The drawing under review shows one solid part. Ordinate dimensions are in mm from its lowest x, y, z. Coordinates: 2 decimals unless noted, no trailing zeros. Loops run counter-clockwise (first coordinate to the right, second up) from the corner with the lowest first, then second, coordinate; pieces in that order, holes last. Notation, with made-up numbers: M -35,-25 L -24,-25 A23 ccw -24,-4 Z; hole C 3,40.25 d5. An arc over 180 degrees is marked long. Put each result on its own line as item: value.
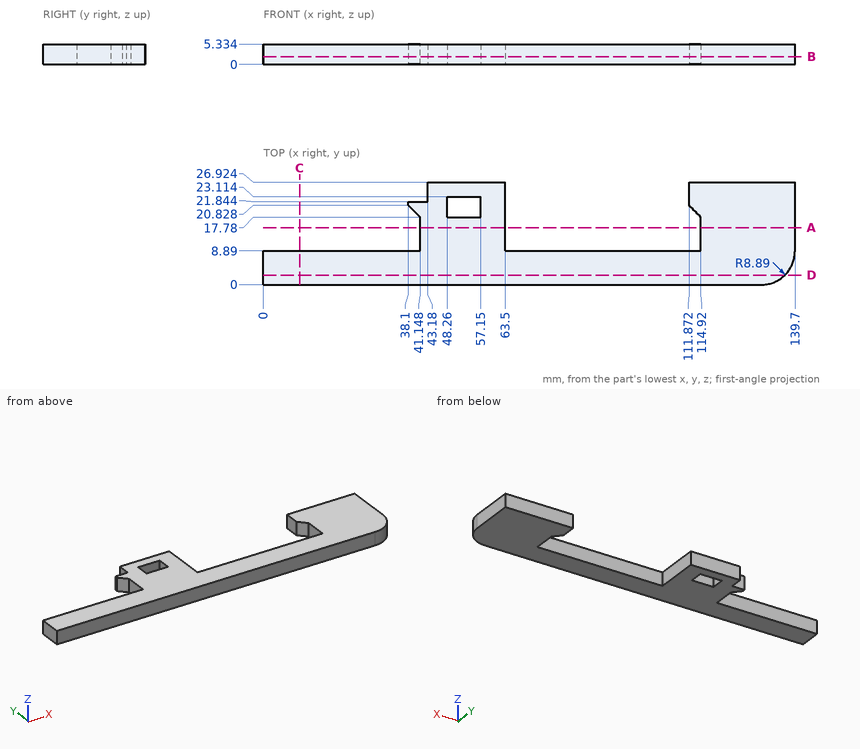
(1) Add section A-A (y = 15). Write out the cut boundary in (x, z), plus the area to 3 significant figures.
Determined:
outline: M 41.15,0 L 63.5,0 L 63.5,5.33 L 41.15,5.33 Z; M 114.92,0 L 139.7,0 L 139.7,5.33 L 114.92,5.33 Z
area: 251 mm^2
(2) For pin 1 (2.5 mm diameter, centred on x = 40.5, z = 3, fed in from +Y); pin 2 (1.6 mm diameter, centred on x = 102, z = 3, fed in from +Y); pin 3 (0.5 mm diameter, centred on y = 21.5, z = 3, fed in from -X), all flat-tipped, find the tip position at first contact; note any pin that passes through.
Determined:
pin 1: stops at y = 21.84
pin 2: stops at y = 8.89
pin 3: stops at x = 38.1
(3) Add section B-B (z = 2). Write out the cut boundary in (x, y), plus the area to 3 significant figures.
Determined:
outline: M 0,0 L 130.81,0 A8.89 ccw 139.7,8.89 L 139.7,26.92 L 111.87,26.92 L 111.87,20.83 L 114.92,17.78 L 114.92,8.89 L 63.5,8.89 L 63.5,26.92 L 43.18,26.92 L 43.18,21.84 L 38.1,21.84 L 38.1,20.83 L 41.15,17.78 L 41.15,8.89 L 0,8.89 Z; hole M 48.26,17.78 L 57.15,17.78 L 57.15,23.11 L 48.26,23.11 Z
area: 2,050 mm^2
(4) Add section C-C (x = 9.5). Write out the cut boundary in (y, z).
Determined:
outline: M 0,0 L 8.89,0 L 8.89,5.33 L 0,5.33 Z
(5) Wall thickness on line 1 along X through (y, z) = (21.5, 1.9); line 2 along X through (y, z) = (26, 2); line 3 along X through (y, z) = (9.25, 4.5): over which ranges is each line inside the solid? List them lowest first. Write a range as [from, to].
Determined:
line 1: x = [38.1, 48.26], [57.15, 63.5], [111.87, 139.7]
line 2: x = [43.18, 63.5], [111.87, 139.7]
line 3: x = [41.15, 63.5], [114.92, 139.7]
(6) Add section D-D (y = 2.5). Write out the cut boundary in (x, z), plus the area to 3 significant figures.
Determined:
outline: M 0,0 L 136.99,0 L 136.99,5.33 L 0,5.33 Z
area: 731 mm^2
